Drawing for the job (mm, zero at the part's lowest x, y, z). A direction names the side the tool comes from. Coordinates: 2 decimals unless noted, no trailing zeros. Write each loop counter-clockwise with the first axis right and the second up, starting at its lowest first coordinate (ties: lowest second). Pieces come first, ordered by that corner, then holes. Notation, with made-up numbers: (13, -9) - (39, -9) arc R12 cw to (39, 5) - close; hole circle Ø6 at (82.5, 84.5). An arc over 180 degrees is marked (long way). Write each question's results on one line, items separated by ' | '.
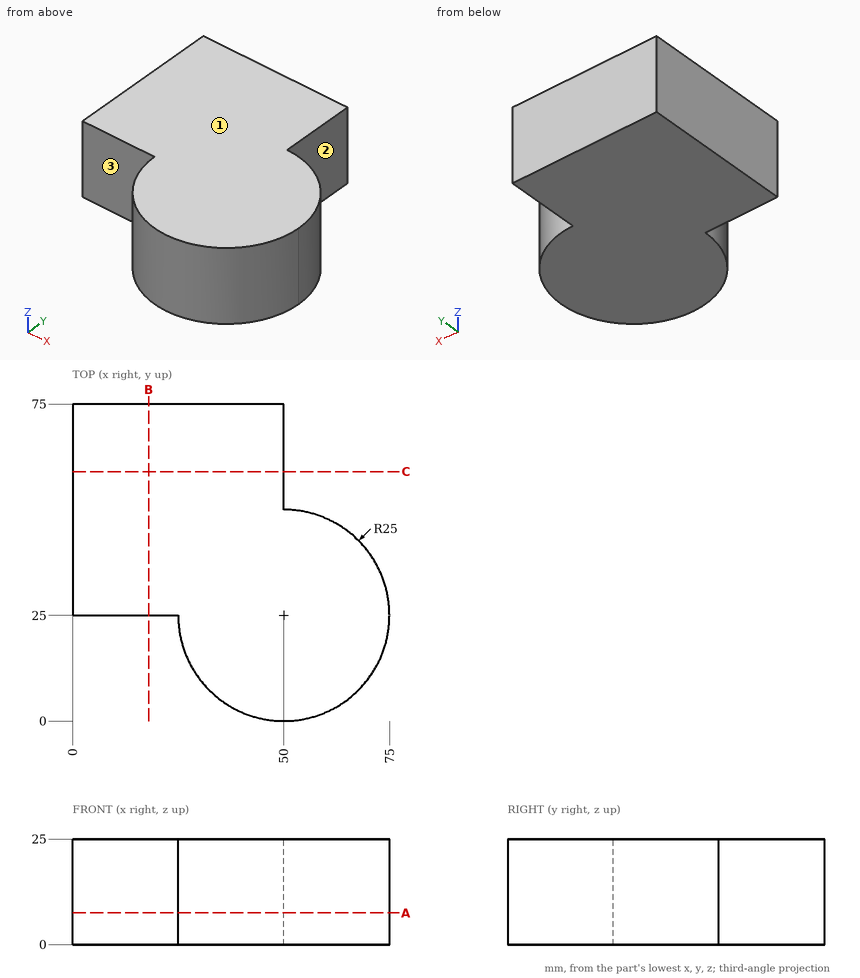
(1) 3-axis set-ups, long thin cutter, end or side, ignore diameter. For the marked faces 1, 2 and 3: which of +Z, -Z, +X, -X, +Y, -Y reach the whole face in a straight line?
Return value:
face 1: +Z, +X, -X, +Y, -Y | face 2: +Z, -Z, +X, +Y | face 3: +Z, -Z, -X, -Y
(2) Flat gauge pins, fed straight in: P1, Ø8, axis at y = 33, z = 18.5, coming from the -X side; P2, Ø1, axis at y = 35, z = 4.5, coming from the +X side; P3, Ø1.5, axis at y = 63.5, z = 5, coming from the +X side; P4, Ø5, axis at y = 19, z = 11.5, coming from the +X side. Where does each tip first touch, or does it go through?
Return value:
P1: stops at x = 0 | P2: stops at x = 73.12 | P3: stops at x = 50 | P4: stops at x = 74.75
(3) Saw through at A-A on z = 7.5. Write the cut outline in (x, y).
Return value:
outline: (0, 25) - (25, 25) arc R25 ccw (long way) to (50, 50) - (50, 75) - (0, 75) - close
(4) Saw through at C-C on y = 59. Write the cut outline in (x, z).
Return value:
outline: (0, 0) - (50, 0) - (50, 25) - (0, 25) - close
(5) Wall check: line 1 (Y direction, x = 7, z = 8); line 2 (X direction, y = 69, z = 11.75); line 3 (X direction, y = 13, z = 7). Give the ranges that are in metal, low to high. Write a range as from..to.
Return value:
line 1: y = 25..75 | line 2: x = 0..50 | line 3: x = 28.07..71.93
(6) Saw through at B-B on x = 18. Write the cut outline in (y, z).
Return value:
outline: (25, 0) - (75, 0) - (75, 25) - (25, 25) - close
